Here's how the part is built. I have some questions about the finished solid (model axes, mm). A direction names the side the tool comes from. Round coordinates to 2 decimals unless told otherwise and drop trailing zeros. Loops run counter-clockwise (first coordinate to the right, second up) from the corner with the lowest first, then second, coordinate; pieces in that order, holes last. Notation, with made-up numbers: M -32.5,82.25 L 4.5,82.25 A19 ccw 4.5,106.25 Z; hole C 14.5,-21.5 d4. An arc over 180 degrees is marked long. Use a Markdown table: item, result.
from build123d import *

# Parameters (mm, degrees)
SKETCH_1_R      = 30
SKETCH_1_R_2    = 1.5
EXTRUDE_1_DEPTH = 3


with BuildPart() as part:
    # 草图1 → 凸台-拉伸1 (new body)
    with BuildSketch(Plane(origin=(0, 0, 0), x_dir=(1, 0, 0), z_dir=(0, 1, 0))):
        Circle(SKETCH_1_R)
        with Locations((-12.6, 12.6)):
            Circle(SKETCH_1_R_2, mode=Mode.SUBTRACT)
        with Locations((12.6, 12.6)):
            Circle(SKETCH_1_R_2, mode=Mode.SUBTRACT)
        with Locations((12.6, -12.6)):
            Circle(SKETCH_1_R_2, mode=Mode.SUBTRACT)
        with Locations((-12.6, -12.6)):
            Circle(SKETCH_1_R_2, mode=Mode.SUBTRACT)
    extrude(amount=EXTRUDE_1_DEPTH)

    # 草图3 → 旋转1 (revolve)
    with BuildSketch(Plane(origin=(0, 0, 0), x_dir=(0, 0, -1), z_dir=(1, 0, 0))):
        with BuildLine():
            Line((0, -22.5), (0, 0))
            Line((0, 0), (22.5, 0))
            ThreePointArc((22.5, 0), (15.909902577, -15.909902577), (0, -22.5))
        make_face()
    revolve(axis=Axis((0, 15, 0), (0, 1, 0)))


solid = part.part
1. Imagine slicing it at B-B, the plane z = 0. Write out the boundary of the cut face in (x, y), then the cut area to 3 significant figures.
Answer sheet:
| item | result |
|---|---|
| outline | M -30,0 L -22.5,0 A22.5 ccw 22.5,0 L 30,0 L 30,3 L -30,3 Z |
| area | 975 mm2 |
2. Imagine slicing it at C-C, the plane z = 12.6. Write out the boundary of the cut face in (x, y), then the cut area to 3 significant figures.
Answer sheet:
| item | result |
|---|---|
| outline | M -27.23,0 L -18.64,0 A18.64 ccw 18.64,0 L 27.23,0 L 27.23,3 L 14.1,3 L 14.1,0 L 11.1,0 L 11.1,3 L -11.1,3 L -11.1,0 L -14.1,0 L -14.1,3 L -27.23,3 Z |
| area | 691 mm2 |
3. Imagine slicing it at A-A, the plane x = 0. Write out the boundary of the cut face in (y, z), then the cut area to 3 significant figures.
Answer sheet:
| item | result |
|---|---|
| outline | M 0,-30 L 3,-30 L 3,30 L 0,30 L 0,22.5 A22.5 ccw 0,-22.5 Z |
| area | 975 mm2 |
4. Which directions (+Z, -Z, +X, -X, +Y, -Y) give clear straight access to the entire face, cutting with the end or side of a thin tool? Please do faces 1 (the face through (13, 0, -13)), 2 (the face through (0, 3, 0)).
Answer sheet:
| item | result |
|---|---|
| face 1 | +Y |
| face 2 | +Z, -Z, +X, -X, +Y |
5. Imagine slicing it at D-D, the plane y = -14. Write out the boundary of the cut face in (x, z), then the cut area to 3 significant figures.
Answer sheet:
| item | result |
|---|---|
| outline | C 0,0 d35.23 |
| area | 975 mm2 |
6. For pin 1 Ø1.5 at (x, z) = (12.5, -12.5) entering from +Y; pin 2 Ø12 at (x, z) = (-8.5, 9) entering from -Y; pin 3 Ø2 at (x, y) = (4, -20) entering from +Z; pin 4 Ø1 at (x, z) = (-19, 24) entering from +Y, each with a flat end and sliding along its axis, tell me the tip position at first contact or that it passes through.
Answer sheet:
| item | result |
|---|---|
| pin 1 | y = 0 |
| pin 2 | y = -21.58 |
| pin 3 | z = 11.4 |
| pin 4 | through |
7. I need wall thicknesses on probe 1 along Z at (x, y) = (-12.6, 1.9); probe 2 along Y at (x, z) = (-25.5, 13). Which ranges of each line are inside material? Lowest first, please. Write a range as from..to.
Answer sheet:
| item | result |
|---|---|
| probe 1 | -27.23..-14.1, -11.1..11.1, 14.1..27.23 |
| probe 2 | 0..3 |
8. We'd pull the mould along X, two halves only. Please class faces 3 (the face through (4.3, 0, -22.4)), 4 (the face through (-13, 0, 13)), 5 (the face through (-29.97, 1.48, -1.32)): +X half, -X half, draft (parallel to the pull), parting line (faces both ways), or undercut.
Answer sheet:
| item | result |
|---|---|
| face 3 | draft |
| face 4 | undercut |
| face 5 | parting line |
